Build history of the part. All positions in model axes, mm. Face numbers are marked on the shaded views. A direction names the side the tool comes from. Round coordinates to 2 decimals unless told otherwise and drop trailing zeros. Loops run counter-clockwise (first coordinate to the right, second up) from the corner with the lowest first, then second, coordinate; pieces in that order, holes last. Notation, with made-up numbers: (18.25, -20) -> (49.25, -20) arc R12 ccw to (49.25, -5) -> close; hole circle Ø7 at (42, -8). An arc over 180 degrees is marked (long way). Put each result on its own line as item: value. Start each with the question number.
Item 1: Drill centre lines: probe 1 along X at (y, z) = (0.75, 0); probe 2 along X at (y, z) = (2.05, -10); probe 3 along X at (y, z) = (0.4, 6). Where is each one in solid material? Low to high. Write a range as [from, to].
Item 2: Flat gauge pins, fed straight in: pin 1 Ø0.8 at (y, z) = (1, 9.5) entering from +X; pin 2 Ø1.5 at (x, y) = (-5, 1.5) entering from +Z; pin 3 Ø1.5 at (y, z) = (1, 6) entering from +X. Where does each tip first touch, or does it go through?
Item 3: Cut at A-A, the plane x = 0. List the corners of the cut face in (y, z).
Item 4: Cut at D-D, the plane x = -5.5. List the corners of the cut face in (y, z), plus the area to 3 significant figures.
Item 5: Cut at C-C, the plane z = 5. List the corners of the cut face in (x, y), plus the area to 3 significant figures.
Item 6: Cut at B-B, the plane z = 0. List the corners of the cut face in (x, y).
Item 7: Tool access for the marked faces 1, 2, 3, 4 and 5: list every direction of +Z, -Z, +X, -X, +Y, -Y with a clear straight run to the whole face (end or side of a thin tool).
Item 8: Pull direction Z, two halves, no side cores. Call the marked faces 6, 7, 8 and 9: +Z half, -Z half, draft (parallel to the pull), parting line (faces both ways), or undercut.
```python
from build123d import *

# Parameters (mm, degrees)
SKETCH1_W           = 14.2
SKETCH1_H           = 14.2
BOSS_EXTRUDE1_DEPTH = 3
SKETCH2_R           = 0.8
CUT_EXTRUDE1_DEPTH  = 17.552945357
FILLET1_R           = 1


with BuildPart() as part:
    # Sketch1 → Boss-Extrude1 (new body)
    with BuildSketch(Plane(origin=(0, 0, 0), x_dir=(1, 0, 0), z_dir=(0, 1, 0))):
        with BuildLine():
            Line((-9, 2), (-8.3, 2))
            Line((-8.3, 2), (-8.3, 8.3))
            Line((-8.3, 8.3), (-2, 8.3))
            Line((-2, 8.3), (-2, 10))
            ThreePointArc((-2, 10), (0, 12), (2, 10))
            Line((2, 10), (2, 8.3))
            Line((2, 8.3), (8.3, 8.3))
            Line((8.3, 8.3), (8.3, 2))
            Line((8.3, 2), (9, 2))
            ThreePointArc((9, 2), (11, 0), (9, -2))
            Line((9, -2), (8.3, -2))
            Line((8.3, -2), (8.3, -8.3))
            Line((8.3, -8.3), (2, -8.3))
            Line((2, -8.3), (2, -10))
            ThreePointArc((2, -10), (0, -12), (-2, -10))
            Line((-2, -10), (-2, -8.3))
            Line((-2, -8.3), (-8.3, -8.3))
            Line((-8.3, -8.3), (-8.3, -2))
            Line((-8.3, -2), (-9, -2))
            ThreePointArc((-9, -2), (-11, 0), (-9, 2))
        make_face()
        Rectangle(SKETCH1_W, SKETCH1_H, mode=Mode.SUBTRACT)
    extrude(amount=BOSS_EXTRUDE1_DEPTH)

    # Sketch2 → Cut-Extrude1 (cut, through all)
    with BuildSketch(Plane(origin=(0, 3, 0), x_dir=(1, 0, 0), z_dir=(0, 1, 0))):
        with Locations(Location((0, 10, 0), (0, 0, 270))):
            Circle(SKETCH2_R)
        with Locations(Location((9, 0, 0), (0, 0, 270))):
            Circle(SKETCH2_R)
        with Locations(Location((0, -10, 0), (0, 0, 270))):
            Circle(SKETCH2_R)
        with Locations(Location((-9, 0, 0), (0, 0, 270))):
            Circle(SKETCH2_R)
    extrude(amount=-CUT_EXTRUDE1_DEPTH, mode=Mode.SUBTRACT)

    # Fillet1
    fillet1_edges = [part.edges().sort_by_distance(p)[0] for p in [
        (-2, 1.5, 8.3),
        (2, 1.5, 8.3),
        (8.3, 1.5, 2),
        (8.3, 1.5, -2),
        (2, 1.5, -8.3),
        (-2, 1.5, -8.3),
        (-8.3, 1.5, -2),
        (-8.3, 1.5, 2),
    ]]
    fillet(fillet1_edges, radius=FILLET1_R)


solid = part.part
```
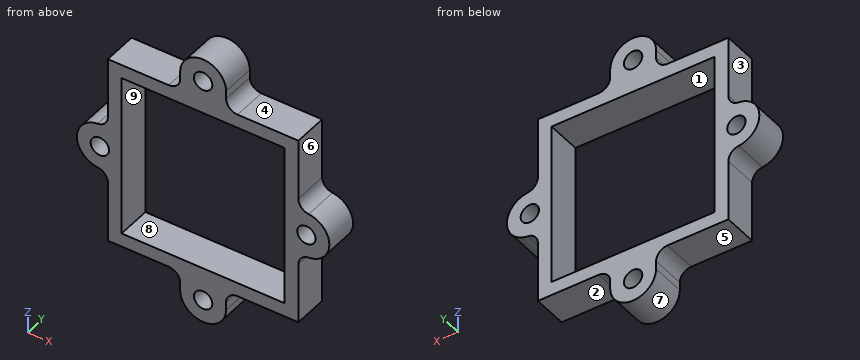
Reply:
1. probe 1: x = [-11, -9.8], [-8.2, -7.1], [7.1, 8.2], [9.8, 11]
1. probe 2: x = [-2, -0.8], [0.8, 2]
1. probe 3: x = [-8.3, -7.1], [7.1, 8.3]
2. pin 1: stops at x = 2.02
2. pin 2: stops at z = 8.3
2. pin 3: stops at x = 8.3
3. outline: (0, -12) -> (3, -12) -> (3, -10.8) -> (0, -10.8) -> close; (0, -9.2) -> (3, -9.2) -> (3, -7.1) -> (0, -7.1) -> close; (0, 7.1) -> (3, 7.1) -> (3, 9.2) -> (0, 9.2) -> close; (0, 10.8) -> (3, 10.8) -> (3, 12) -> (0, 12) -> close
4. outline: (0, -8.3) -> (3, -8.3) -> (3, -7.1) -> (0, -7.1) -> close; (0, 7.1) -> (3, 7.1) -> (3, 8.3) -> (0, 8.3) -> close
4. area: 7.20 mm^2
5. outline: (-8.3, 0) -> (-7.1, 0) -> (-7.1, 3) -> (-8.3, 3) -> close; (7.1, 0) -> (8.3, 0) -> (8.3, 3) -> (7.1, 3) -> close
5. area: 7.20 mm^2
6. outline: (-11, 0) -> (-9.8, 0) -> (-9.8, 3) -> (-11, 3) -> close; (-8.2, 0) -> (-7.1, 0) -> (-7.1, 3) -> (-8.2, 3) -> close; (7.1, 0) -> (8.2, 0) -> (8.2, 3) -> (7.1, 3) -> close; (9.8, 0) -> (11, 0) -> (11, 3) -> (9.8, 3) -> close
7. face 1: +Y, -Y
7. face 2: -Z, +X, +Y, -Y
7. face 3: +Z, -X, +Y, -Y
7. face 4: +Z, +X, +Y, -Y
7. face 5: -Z, -X, +Y, -Y
8. face 6: draft
8. face 7: -Z half
8. face 8: undercut
8. face 9: undercut
